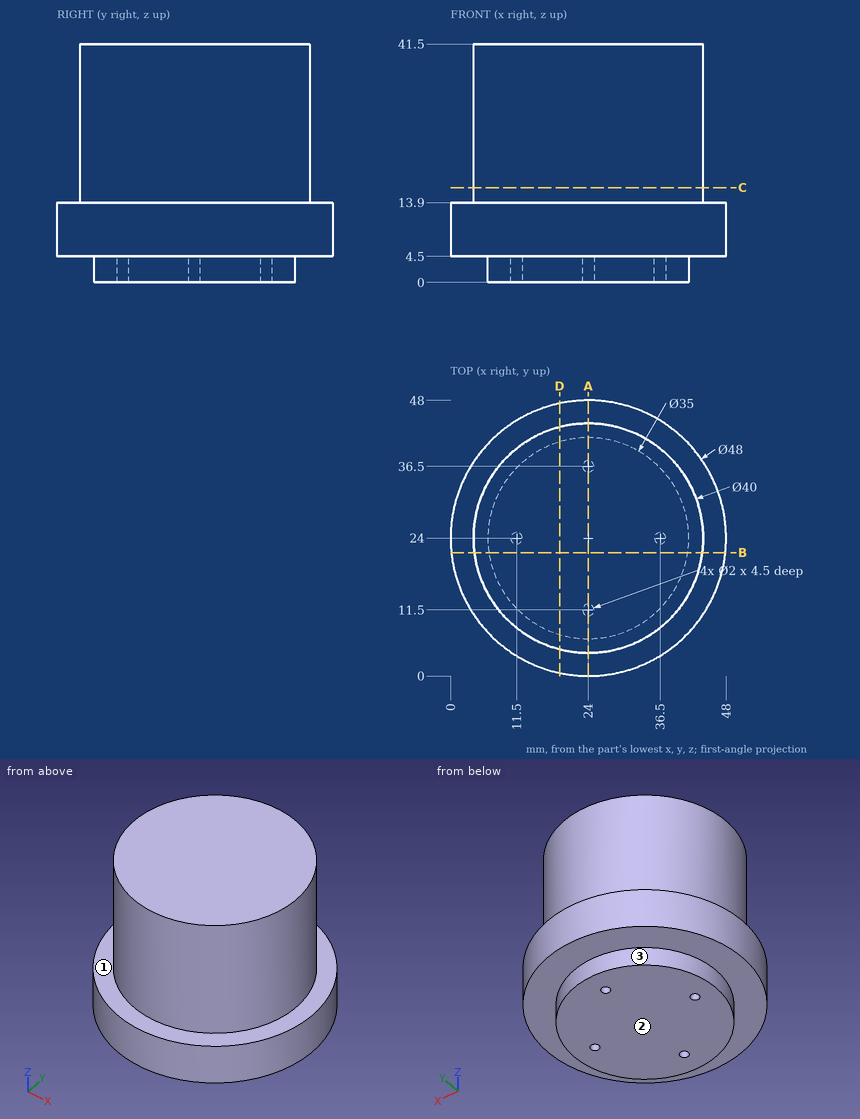
Could you check a few things on this drawing? It's one solid part, dimensions in mm from its lowest x, y, z. A direction names the side the tool comes from. Coordinates: 2 decimals unless noted, no trailing zeros. Write each loop counter-clockwise with the first axis right and the second up, starting at its lowest first coordinate (ties: lowest second). Pieces come first, ordered by that corner, then holes.
Q1. Imagine slicing it at B-B, the plane y = 21.5. List the corners of the cut face in (x, z) for me.
Results found:
outline: (0.13, 4.5) - (6.68, 4.5) - (6.68, 0) - (41.32, 0) - (41.32, 4.5) - (47.87, 4.5) - (47.87, 13.9) - (43.84, 13.9) - (43.84, 41.5) - (4.16, 41.5) - (4.16, 13.9) - (0.13, 13.9) - close
Q2. Please list where these lines run through material, in increasing order: L1, parallel to Y at x = 24, z = 2; L2, parallel to Z at x = 8, y = 35.5; L3, parallel to Y at x = 36.5, z = 3.5.
Results found:
L1: y = 6.5 to 10.5, 12.5 to 35.5, 37.5 to 41.5
L2: z = 4.5 to 41.5
L3: y = 11.75 to 23, 25 to 36.25
Q3. Which directions (+Z, -Z, +X, -X, +Y, -Y) give clear straight access to the entire face, cutting with the end or side of a thin tool? Please do the marked faces 1, 2 and 3.
Results found:
face 1: +Z
face 2: -Z, +X, -X, +Y, -Y
face 3: -Z
Q4. Imagine slicing it at D-D, the plane x = 19. List the corners of the cut face in (y, z) for me, plus the area to 3 significant figures.
Results found:
outline: (0.53, 4.5) - (7.23, 4.5) - (7.23, 0) - (40.77, 0) - (40.77, 4.5) - (47.47, 4.5) - (47.47, 13.9) - (43.36, 13.9) - (43.36, 41.5) - (4.64, 41.5) - (4.64, 13.9) - (0.53, 13.9) - close
area: 1,660 mm2
Q5. For P1, Ø4, axis at x = 5, z = 32.5, coming from the +Y side; P2, Ø4, axis at x = 38.5, y = 5.5, coming from the +Z side; P3, Ø10, axis at y = 5, z = 14, coming from the +X side, each with a flat end and sliding along its axis, tell me the tip position at first contact or that it passes through.
Results found:
P1: stops at y = 34.54
P2: stops at z = 13.9
P3: stops at x = 43.49
Q6. Imagine slicing it at C-C, the plane z = 16.5. List the corners of the cut face in (x, y) for me.
Results found:
outline: circle Ø40 at (24, 24)
Q7. Imagine slicing it at A-A, the plane x = 24. List the corners of the cut face in (y, z) for me.
Results found:
outline: (0, 4.5) - (6.5, 4.5) - (6.5, 0) - (10.5, 0) - (10.5, 4.5) - (12.5, 4.5) - (12.5, 0) - (35.5, 0) - (35.5, 4.5) - (37.5, 4.5) - (37.5, 0) - (41.5, 0) - (41.5, 4.5) - (48, 4.5) - (48, 13.9) - (44, 13.9) - (44, 41.5) - (4, 41.5) - (4, 13.9) - (0, 13.9) - close
